```python
from build123d import *
from OCP.BRepFilletAPI import BRepFilletAPI_MakeChamfer

# Parameters (mm, degrees)
SKETCH_1_W                  = 82
SKETCH_1_H                  = 63.5
EXTRUDE_1_DEPTH             = 16
CUT_EXTRUDE_1_DEPTH         = 105.939268151
SKETCH_15_W                 = 23.6
SKETCH_15_H                 = 14.711451884
CUT_EXTRUDE_4_DEPTH         = 7
SKETCH_16_W                 = 23.6
SKETCH_16_H                 = 10.67
CUT_EXTRUDE_5_DEPTH         = 9
SKETCH_17_R                 = 2.5
CUT_EXTRUDE_6_DEPTH         = 8
M4X0_72_D                   = 3.3
M4X0_72_DEPTH               = 10
M4X0_72_TIP                 = 0.991420021
CUT_EXTRUDE_7_DEPTH         = 4
SKETCH_26_R                 = 3.25
CUT_EXTRUDE_8_DEPTH         = 38
HOLE_WIZARD_M41_D           = 4.5
HOLE_WIZARD_M41_CBORE_D     = 8
HOLE_WIZARD_M41_CBORE_DEPTH = 4
CHAMFER_2_SIZE              = 1
CHAMFER_2_SIZE2             = 2
CUT_EXTRUDE_12_DEPTH        = 10.6
FILLET_1_R                  = 3
M3X0_51_D                   = 2.5


with BuildPart() as part:
    # Эскиз1 → Бобышка-Вытянуть1 (new body)
    with BuildSketch(Plane.XY):
        with Locations((41, -31.75)):
            Rectangle(SKETCH_1_W, SKETCH_1_H)
    extrude(amount=EXTRUDE_1_DEPTH)

    # Эскиз2 → Вырез-Вытянуть1 (cut, through all)
    with BuildSketch(Plane.ZY):
        Polygon((9, -10.67), (16, -14.711451884), (16, -48.788548116), (9, -52.83), align=None)
    extrude(amount=-CUT_EXTRUDE_1_DEPTH, mode=Mode.SUBTRACT)

    # Эскиз15 → Вырез-Вытянуть4 (cut)
    with BuildSketch(Plane.XY.offset(16)):
        with Locations((41, -56.144274058)):
            Rectangle(SKETCH_15_W, SKETCH_15_H)
    extrude(amount=-CUT_EXTRUDE_4_DEPTH, mode=Mode.SUBTRACT)

    # Эскиз16 → Вырез-Вытянуть5 (cut)
    with BuildSketch(Plane.XY.offset(9)):
        with Locations((41, -58.165)):
            Rectangle(SKETCH_16_W, SKETCH_16_H)
    extrude(amount=-CUT_EXTRUDE_5_DEPTH, mode=Mode.SUBTRACT)

    # Эскиз17 → Вырез-Вытянуть6 (cut)
    with BuildSketch(Plane.XZ.offset(52.83)):
        with Locations(Location((33.5, 5, 0), (0, 0, 270))):
            Circle(SKETCH_17_R)
        with Locations(Location((48.5, 5, 0), (0, 0, 90))):
            Circle(SKETCH_17_R)
    extrude(amount=-CUT_EXTRUDE_6_DEPTH, mode=Mode.SUBTRACT)

    # Отверстие обработанное метчиком M4x0.72
    with Locations(Plane(origin=(0, -52.83, 0), x_dir=(-1, 0, 0), z_dir=(0, -1, 0))):
        with Locations((-41, -5)):
            Hole(M4X0_72_D / 2, depth=M4X0_72_DEPTH)
            with Locations((0, 0, -(M4X0_72_DEPTH + M4X0_72_TIP / 2))):  # 118° drill point
                Cone(0, M4X0_72_D / 2, M4X0_72_TIP, mode=Mode.SUBTRACT)

    # Эскиз25 → Вырез-Вытянуть7 (cut)
    with BuildSketch(Plane.XY.offset(9)):
        with BuildLine():
            Line((44.1, -18.711451884), (44.1, -25.711451884))
            ThreePointArc((44.1, -25.711451884), (41, -28.811451884), (37.9, -25.711451884))
            Line((37.9, -25.711451884), (37.9, -18.711451884))
            ThreePointArc((37.9, -18.711451884), (41, -15.611451884), (44.1, -18.711451884))
        make_face()
    extrude(amount=-CUT_EXTRUDE_7_DEPTH, mode=Mode.SUBTRACT)

    # Эскиз26 → Вырез-Вытянуть8 (cut)
    with BuildSketch(Plane(origin=(0, 0, 0), x_dir=(1, 0, 0), z_dir=(0, 1, 0))):
        with Locations(Location((41, -4.5, 0), (0, 0, 270))):
            Circle(SKETCH_26_R)
    extrude(amount=-CUT_EXTRUDE_8_DEPTH, mode=Mode.SUBTRACT)

    # Цековка для винта с внутренним шестигранником M41 (through all)
    with Locations(Plane(origin=(30.759227947, 26.793365177, 16), x_dir=(-1, 0, 0), z_dir=(0, 0, 1))):
        with Locations((-46.240772053, 31.793365177), (-46.240772053, 85.293365177), (25.759227947, 85.293365177), (25.759227947, 31.793365177)):
            CounterBoreHole(HOLE_WIZARD_M41_D / 2, HOLE_WIZARD_M41_CBORE_D / 2, HOLE_WIZARD_M41_CBORE_DEPTH)

    # Фаска2: one chamfer whose edges measure the first distance from different faces: ONE call of the kernel's chamfer builder (chamfer() names one face for all edges)
    chamfer_2_edges_1 = [part.edges().sort_by_distance(p)[0] for p in [
        (41, -14.711451884, 16),
    ]]
    chamfer_2_side_1 = [part.faces().sort_by_distance(p)[0] for p in [
        (41, -7.569889145, 16),
    ]]
    chamfer_2_edges_2 = [part.edges().sort_by_distance(p)[0] for p in [
        (67.4, -48.788548116, 16),
    ]]
    chamfer_2_side_2 = [part.faces().sort_by_distance(p)[0] for p in [
        (66.127821531, -55.832096576, 16),
    ]]
    chamfer_2_edges_3 = [part.edges().sort_by_distance(p)[0] for p in [
        (14.6, -48.788548116, 16),
    ]]
    chamfer_2_side_3 = [part.faces().sort_by_distance(p)[0] for p in [
        (15.872178469, -55.832096576, 16),
    ]]
    chamfer_2 = BRepFilletAPI_MakeChamfer(part.part.solid().wrapped)
    for e in chamfer_2_edges_1:
        chamfer_2.Add(CHAMFER_2_SIZE, CHAMFER_2_SIZE2, e.wrapped, chamfer_2_side_1[0].wrapped)  # the first distance lies on this face
    for e in chamfer_2_edges_2:
        chamfer_2.Add(CHAMFER_2_SIZE, CHAMFER_2_SIZE2, e.wrapped, chamfer_2_side_2[0].wrapped)  # the first distance lies on this face
    for e in chamfer_2_edges_3:
        chamfer_2.Add(CHAMFER_2_SIZE, CHAMFER_2_SIZE2, e.wrapped, chamfer_2_side_3[0].wrapped)  # the first distance lies on this face
    add(Compound.cast(chamfer_2.Shape()), mode=Mode.REPLACE)

    # Эскиз32 → Вырез-Вытянуть12 (cut)
    with BuildSketch(Plane.XZ.offset(63.5)):
        with BuildLine():
            Line((52.7, -0.2), (52.7, 3.7))
            Line((52.7, 3.7), (58.5, 3.7))
            ThreePointArc((58.5, 3.7), (62.8, 8), (58.5, 12.3))
            Line((58.5, 12.3), (52.7, 12.3))
            Line((52.7, 12.3), (52.7, 16.2))
            Line((52.7, 16.2), (29.3, 16.2))
            Line((29.3, 16.2), (29.3, 12.3))
            Line((29.3, 12.3), (23.5, 12.3))
            ThreePointArc((23.5, 12.3), (19.2, 8), (23.5, 3.7))
            Line((23.5, 3.7), (29.3, 3.7))
            Line((29.3, 3.7), (29.3, -0.2))
            Line((29.3, -0.2), (52.7, -0.2))
        make_face()
    extrude(amount=-CUT_EXTRUDE_12_DEPTH, mode=Mode.SUBTRACT)

    # Скругление1
    fillet_1_edges = [part.edges().sort_by_distance(p)[0] for p in [
        (52.8, -58.2, 3.7),
        (52.8, -58.2, 12.3),
        (29.2, -58.2, 12.3),
        (29.2, -58.2, 3.7),
    ]]
    fillet(fillet_1_edges, radius=FILLET_1_R)

    # Отверстие обработанное метчиком M3x0.51 (through all)
    with Locations(Plane(origin=(0, 0, 0), x_dir=(-1, 0, 0), z_dir=(0, 0, -1))):
        with Locations((-26, -44.75), (-26, -18.75), (-56, -18.75), (-56, -44.75)):
            Hole(M3X0_51_D / 2)


solid = part.part
```
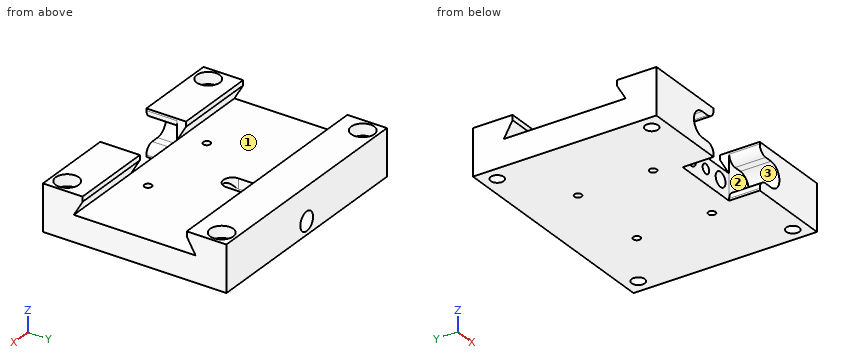
Work out the finished part from the listing and answer in its coordinate system (mm). Face numbers are marked on the shaded views. Coordinates: 2 decimals unless noted, no trailing zeros. Order: outer loops, then holes, each group sorted by start corner. A loop starts at its lowest first (then second) coordinate and runs counter-clockwise, first axis right, second up. Notation, with made-up numbers: M 82.5,80.25 L 132.5,80.25 A16 cw 132.5,85.25 Z; hole C 77.5,-29 d9. An arc over 180 degrees is marked long. Use CSV: the item, a comma, the result in double quotes.
1) Section A-A on y = -6 is taken. Write down the section's boundary in (x, z).
Worked out:
outline,"M 0,0 L 2.98,0 L 2.98,12 L 1.13,12 L 1.13,16 L 0,16 Z; M 7.02,0 L 74.98,0 L 74.98,12 L 73.13,12 L 73.13,16 L 8.87,16 L 8.87,12 L 7.02,12 Z; M 79.02,0 L 82,0 L 82,16 L 80.87,16 L 80.87,12 L 79.02,12 Z; hole C 41,4.5 d6.5"
2) Section B-B on x = 77 is taken. Write down the section's boundary in (y, z).
Worked out:
outline,"M -63.5,0 L -60.75,0 L -60.75,12 L -62.5,12 L -62.5,16 L -63.5,16 Z; M -56.25,0 L -7.25,0 L -7.25,12 L -9,12 L -9,16 L -13.71,16 L -13.71,14.27 L -10.67,9 L -52.83,9 L -49.79,14.27 L -49.79,16 L -54.5,16 L -54.5,12 L -56.25,12 Z; M -2.75,0 L 0,0 L 0,16 L -1,16 L -1,12 L -2.75,12 Z"
3) Section D-D on y = -51.5 is taken. Write down the section's boundary in (x, z).
Worked out:
outline,"M 0,0 L 82,0 L 82,9 L 0,9 Z; M 0,11.3 L 29.2,11.3 L 29.2,16 L 0,16 Z; M 52.8,11.3 L 82,11.3 L 82,16 L 52.8,16 Z; hole C 33.5,5 d5; hole C 41,5 d3.3; hole C 48.5,5 d5"
4) Consider line 1 (X direction, y = -49.25, z = 5); line 2 (Y direction, x = 77, z = 4.75); line 3 (Z direction, x = 41, y = -48). Determine where each line is inside the solid, lowest interval first. Write a range as [from, to].
Worked out:
line 1,"x = [0, 31], [36, 39.35], [42.65, 46], [51, 82]"
line 2,"y = [-63.5, -60.75], [-56.25, -7.25], [-2.75, 0]"
line 3,"z = [0, 3.35], [6.65, 9]"
5) Flat-ended cylindrical pins translate along their axes: pin 1 Ø2 at (x, y) = (24.5, -56) entering from -Z; pin 2 Ø6 at (x, y) = (77, -58.5) entering from +Z; pin 3 Ø4 at (x, y) = (56, -18.75) entering from +Z; pin 4 Ø1.5 at (x, y) = (26, -18.75) entering from -Z. Find the tip coordinate at first contact, or state that the pin passes through.
Worked out:
pin 1,"stops at z = 0"
pin 2,"stops at z = 12"
pin 3,"stops at z = 9"
pin 4,"passes through"
6) Section C-C on z = 10.5 is taken. Write down the section's boundary in (x, y), plus the area to 3 significant figures.
Worked out:
outline,"M 0,-63.5 L 20,-63.5 L 20,-52.9 L 29.2,-52.9 L 29.2,-51.96 L 0,-51.96 Z; M 0,-11.54 L 82,-11.54 L 82,0 L 0,0 Z; M 52.8,-52.9 L 62,-52.9 L 62,-63.5 L 82,-63.5 L 82,-51.96 L 52.8,-51.96 Z; hole C 5,-58.5 d4.5; hole C 5,-5 d4.5; hole C 77,-58.5 d4.5; hole C 77,-5 d4.5"
area,"1,360 mm^2"
7) Determine the mould class of the marked faces 1, 2 and 3 for opening direction Y: released by +Y, released by -Y, zero draft, split by the parting line, or undercut.
Worked out:
face 1,"undercut"
face 2,"released by -Y"
face 3,"zero draft"
